```python
from build123d import *

# Parameters (mm, degrees)
F3_DEPTH    = 2
F4_W        = 1
F4_H        = 17.3801295459
F5_DEPTH    = 13.251
F6_R        = 5
F7_T1_DEPTH = 1
F8_T1_DEPTH = 11.6824583655
F9_DEPTH    = 1


# Not quite as in the source:
# - a fillet or chamfer that OpenCascade refuses, or shapes differently, is made with other operations: its cross-section is extruded or revolved along the edge and cut away or added


with BuildPart() as f3:
    # F2 (on line) → F3 (new body)
    with BuildSketch(Plane(origin=(0, -12, 0), x_dir=(-1, 0, 0), z_dir=(0, 1, 0))):
        Polygon((-7.75, 0), (-1.75, 0), (-1.75, 8.5), (-3.25, 8.5), (-3.25, 17.5), (-5.5, 17.5), (-6.3357864376, 17.5), (-7.75, 16.0857864376), align=None)
        Polygon((5.5, 17.5), (3.25, 17.5), (3.25, 8.5), (1.75, 8.5), (1.75, 0), (7.75, 0), (7.75, 16.0857864376), (6.3357864376, 17.5), align=None)
        Polygon((-5.5, 17.5), (-3.25, 17.5), (3.25, 17.5), (5.5, 17.5), (5.5, 34.8801295459), (0, 34.8801295459), (-5.5, 34.8801295459), align=None)
    extrude(amount=F3_DEPTH)

    # F4 (on face) → F5 (cut, through all)
    with BuildSketch(Plane.YZ.offset(5.5)):
        with Locations((-10.5, 26.190064773)):
            Rectangle(F4_W, F4_H)
    extrude(amount=-F5_DEPTH, mode=Mode.SUBTRACT)

    # F6
    f6_edges = [f3.edges().sort_by_distance(p)[0] for p in [
        (5.5, -11.5, 34.88013),
        (-5.5, -11.5, 34.88013),
    ]]
    fillet(f6_edges, radius=F6_R)

    # F7: fillet of radius 1 on 2 edges, made by hand

    # F7_s2 → F7_t1 (join)
    with BuildSketch(Plane.XZ.offset(11)):
        with BuildLine():
            ThreePointArc((5.5, 18.4864248101), (5.7370407736, 17.8399782007), (6.3357864376, 17.5))
            Line((6.3357864376, 17.5), (5.5, 17.5))
            Line((5.5, 17.5), (5.5, 18.4864248101))
        make_face()
        with BuildLine():
            ThreePointArc((-6.3357864376, 17.5), (-5.7370407736, 17.8399782007), (-5.5, 18.4864248101))
            Line((-5.5, 18.4864248101), (-5.5, 17.5))
            Line((-5.5, 17.5), (-6.3357864376, 17.5))
        make_face()
    extrude(amount=F7_T1_DEPTH)

    # F8: fillet of radius 2 on 2 edges, made by hand

    # F8_s2 → F8_t1 (cut)
    with BuildSketch(Plane.XZ.offset(5.1587708172)):
        with BuildLine():
            ThreePointArc((3.25, 8.5), (2.1688611699, 7.7882531983), (1.75, 6.5635083269))
            Line((1.75, 6.5635083269), (1.75, 8.5))
            Line((1.75, 8.5), (3.25, 8.5))
        make_face()
        with BuildLine():
            ThreePointArc((-1.75, 6.5635083269), (-2.1688611699, 7.7882531983), (-3.25, 8.5))
            Line((-3.25, 8.5), (-1.75, 8.5))
            Line((-1.75, 8.5), (-1.75, 6.5635083269))
        make_face()
    extrude(amount=F8_T1_DEPTH, mode=Mode.SUBTRACT)

    # F9 (add): a face of the model
    f9_faces = [f3.faces().sort_by_distance(p)[0] for p in [
        (-5.4458267789, -12, 17.5932359202),
    ]]
    extrude(f9_faces, amount=F9_DEPTH)


solid = f3.part
```
Could you check a few things on this model? Use its own coordinates, in mm. A direction names the side the tool comes from. Give positions to 0.01 mm unless a question says otherwise; leave off trailing zeros. Write each loop counter-clockwise with the first axis right and the second up, starting at its lowest first coordinate (ties: lowest second). Pieces come first, ordered by that corner, then holes. Notation, with made-up numbers: (47, 34.25) - (72, 34.25) arc R27 ccw to (72, 54.25) - close; hole circle Ø2 at (48, 11.5). An arc over 180 degrees is marked (long way). One line per item, written item: value. Start each with the question number.
Item 1: Imagine slicing it at C-C, the plane z = 15.5. List the corners of the cut face in (x, y) for me.
Item 2: Imagine slicing it at D-D, the plane x = -6. List the corners of the cut face in (y, z) for me, and give its area (3 significant figures).
Item 3: If we mould it in two halves opening along X, with no side actions, what happens to faces 5 (the face through (0, -12, 34.88)), 6 (the face through (-1.75, -11, 3)), 7 (the face through (-2.18, -11.48, 7.8)), 8 (the face through (4, -11.99, 33.45))? For each: +X half, -X half, draft (parallel to the pull), parting line (faces both ways), or undercut.
Item 4: Which directions (+Z, -Z, +X, -X, +Y, -Y) give clear straight access to the entire face, cutting with the end or side of a thin tool? Please do faces 1 (the face through (0, -11, 26)), 2 (the face through (3.25, -11, 13)), 3 (the face through (-5.5, -12, 24)), 4 (the face through (5.5, -12, 24)).
Item 5: Imagine slicing it at A-A, the plane z = 4.5. List the corners of the cut face in (x, y) for me.
Item 6: Imagine slicing it at B-B, the plane y = -11.35. List the corners of the cut face in (x, z) for me, and give its area (3 significant figures).
Item 7: I'm going to push a flat-ended pin straight in: pin 1 (0.8 mm diameter, centred on x = -5, y = -10.5, fed in from +Z). Where does the tip first touch, or does it pass through?
Item 8: Please list where these lines run through material, in increasing order: line 1 (X direction, y = -12.05, z = 4); line 2 (X direction, y = -12.9, z = 9); line 3 (Y direction, x = -1.5, z = 27.5). Write a range as from..to.
Geometry says:
1. outline: (-7.75, -13) - (-3.25, -13) - (-3.25, -10) - (-7.75, -10) - close; (3.25, -13) - (7.75, -13) - (7.75, -10) - (3.25, -10) - close
2. outline: (-13, 0) - (-10, 0) - (-10, 17.5) - (-11, 17.5) - (-11, 17.62) - (-13, 17.62) - close
2. area: 52.7 mm^2
3. face 5: draft
3. face 6: undercut
3. face 7: undercut
3. face 8: +X half
4. face 1: +Z, +X, -X, +Y
4. face 2: +Y, -Y
4. face 3: +Z, -X, +Y, -Y
4. face 4: +Z, +X, +Y, -Y
5. outline: (-7.75, -13) - (-1.75, -13) - (-1.75, -10) - (-7.75, -10) - close; (1.75, -13) - (7.75, -13) - (7.75, -10) - (1.75, -10) - close
6. outline: (-7.75, 0) - (-1.75, 0) - (-1.75, 6.56) arc R2 ccw to (-3.25, 8.5) - (-3.25, 17.5) - (3.25, 17.5) - (3.25, 8.5) arc R2 ccw to (1.75, 6.56) - (1.75, 0) - (7.75, 0) - (7.75, 16.09) - (6.34, 17.5) arc R1 cw to (5.5, 18.49) - (5.5, 29.88) arc R5 ccw to (0.5, 34.88) - (-0.5, 34.88) arc R5 ccw to (-5.5, 29.88) - (-5.5, 18.49) arc R1 cw to (-6.34, 17.5) - (-7.75, 16.09) - close
6. area: 360 mm^2
7. pin 1: z = 17.5
8. line 1: -7.75..-1.75, 1.75..7.75
8. line 2: -7.75..-3.25, 3.25..7.75
8. line 3: -13..-11
